Study the drawing (mm; zero at the part's minimum x, y, z) and answer. Give positions to 0.01 mm unless a question says otherwise; leave off trailing zeros. Order: outer loops, then holes, each group sorted by start corner. A loop starts at its lowest first (then second) coordinate and runs counter-clockwise, first axis right, second up.
Item 1: Given pin 1 Ø0.7 at (y, z) = (1.5, 64) entering from +X; pin 2 Ø1.5 at (x, z) = (9.5, 40) entering from +Y; pin 3 Ø1.9 at (y, z) = (14.5, 117.5) entering from -X, each flat-ended and moving along its own axis, determine where each tip first touches the part or whether it passes through.
Item 2: Find the intervals of material crossed by line 1 along Z through (x, y) = (3.5, 7.75); line 2 along Y through (x, z) = (8.5, 66.5); line 3 along Y through (x, z) = (2.5, 83.3), in increasing order.
Item 3: A cutting plane is placed at A-A (z = 53.5). Write down the section's boundary in (x, y).
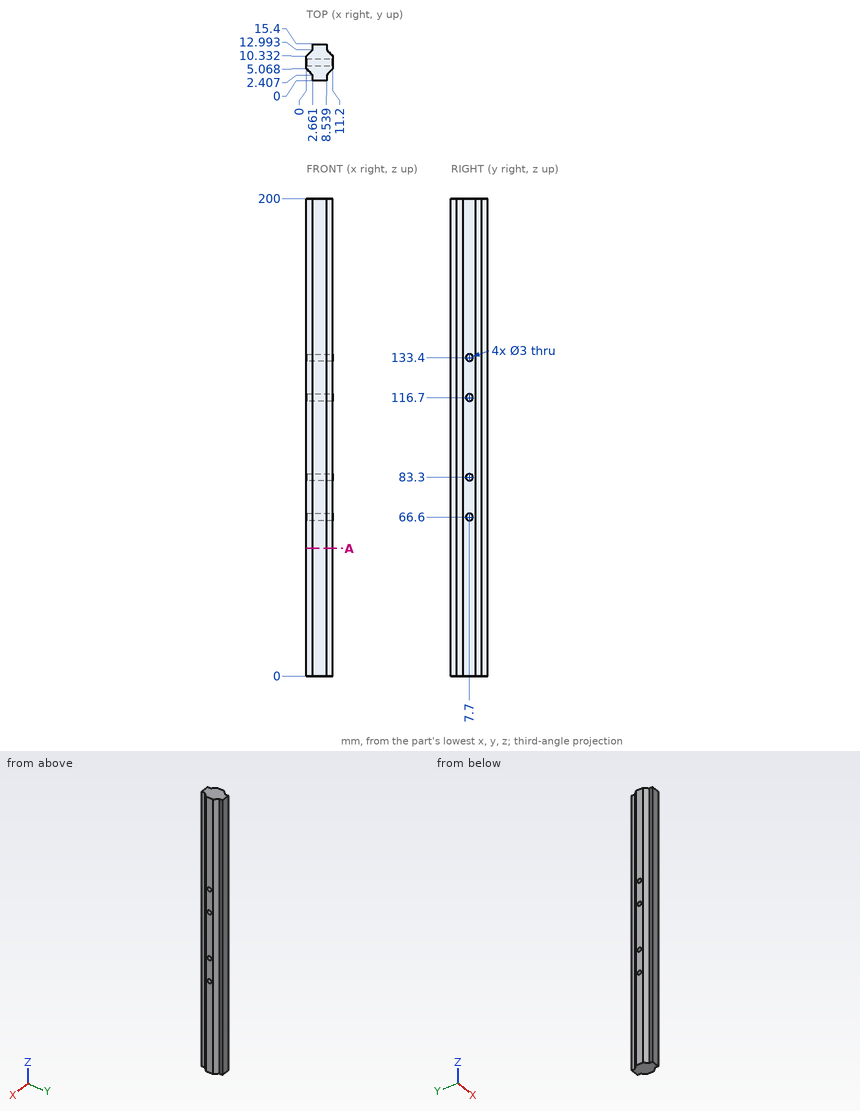
Response values:
1. pin 1: stops at x = 8.54
1. pin 2: stops at y = 12.78
1. pin 3: stops at x = 2.66
2. line 1: z = 0 to 65.1, 68.1 to 81.8, 84.8 to 115.2, 118.2 to 131.9, 134.9 to 200
2. line 2: y = 0 to 6.2, 9.2 to 15.4
2. line 3: y = 2.57 to 6.2, 9.2 to 12.83
3. outline: (0, 5.07) - (2.66, 2.41) - (2.66, 0) - (8.54, 0) - (8.54, 2.41) - (11.2, 5.07) - (11.2, 10.33) - (8.54, 12.99) - (8.54, 15.4) - (2.66, 15.4) - (2.66, 12.99) - (0, 10.33) - close
